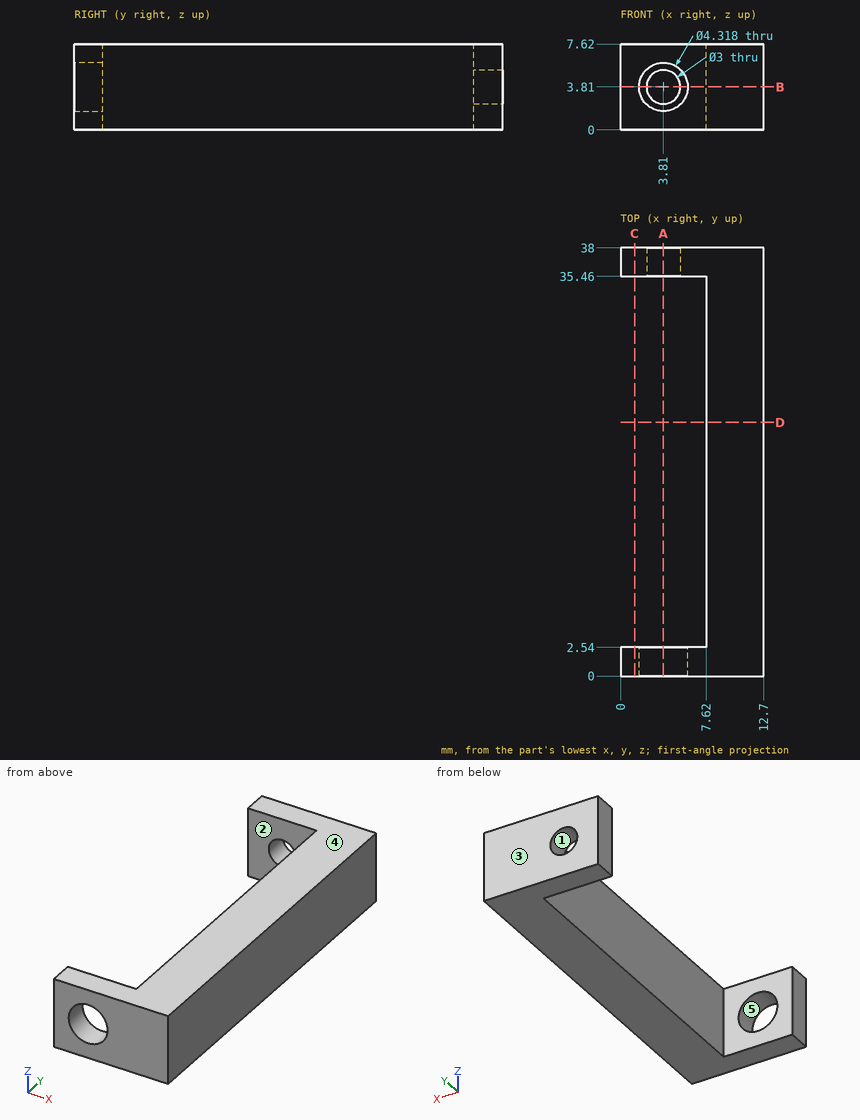
Input: dimensioned drawing with shaded views. Units: mm. Origin: part minimum x, y, z. A direction names the side the tool comes from. Coordinates: 2 decimals unless noted, no trailing zeros. Order: outer loops, then holes, each group sorted by start corner. A loop starts at its lowest first (then second) coordinate and runs counter-clockwise, first axis right, second up.
(1) Material intervals for probe 1 along Y at (x, z) = (0.5, 5.5); probe 2 along X at (y, z) = (1.4, 3.81); probe 3 along X at (y, z) = (31.5, 4), sorted ascending.
(2) Access query for the marked faces 1 and 2. Directions: +Z, -Z, +X, -X, +Y, -Y. A direction counts if a zero-diameter tool reaches every point of the face in a straight line with its end or side. Return the directions, or none.
(3) First-contact query: pin 1 (4 mm diameter, centred on y = 14.5, z = 3.5, fed in from -X); pin 2 (4 mm diameter, centred on x = 3.81, z = 3.81, fed in from -Y). Flat tips, straight axial feed; report the tip coordinate or a pass-through.
(4) Draft query along Z for the marked faces 3, 4 and 5. Return one class per face: pulls with the +Z half, pulls with the -Z half, needs draft (parallel to the pull), parting line crosses it, or undercut.
(5) Section query C-C (x = 1.25). Return the cut outline in (y, z), plus the area to 3 significant figures.
(6) Section query A-A (x = 3.81). Return the cut outline in (y, z).
(7) Section query D-D (y = 22.5). Return the cut outline in (x, z).
(8) Section query B-B (z = 3.81). Return the cut outline in (x, y), plus the area to 3 significant figures.
Solution:
1. probe 1: y = 0 to 2.54, 35.46 to 38
1. probe 2: x = 0 to 1.65, 5.97 to 12.7
1. probe 3: x = 7.62 to 12.7
2. face 1: +Y, -Y
2. face 2: +Z, -Z, -X
3. pin 1: stops at x = 7.62
3. pin 2: stops at y = 35.46
4. face 3: needs draft
4. face 4: pulls with the +Z half
4. face 5: undercut
5. outline: (0, 0) - (2.54, 0) - (2.54, 7.62) - (0, 7.62) - close; (35.46, 0) - (38, 0) - (38, 7.62) - (35.46, 7.62) - close
5. area: 38.7 mm2
6. outline: (0, 0) - (2.54, 0) - (2.54, 1.65) - (0, 1.65) - close; (0, 5.97) - (2.54, 5.97) - (2.54, 7.62) - (0, 7.62) - close; (35.46, 0) - (38, 0) - (38, 2.31) - (35.46, 2.31) - close; (35.46, 5.31) - (38, 5.31) - (38, 7.62) - (35.46, 7.62) - close
7. outline: (7.62, 0) - (12.7, 0) - (12.7, 7.62) - (7.62, 7.62) - close
8. outline: (0, 0) - (1.65, 0) - (1.65, 2.54) - (0, 2.54) - close; (0, 35.46) - (2.31, 35.46) - (2.31, 38) - (0, 38) - close; (5.31, 35.46) - (7.62, 35.46) - (7.62, 2.54) - (5.97, 2.54) - (5.97, 0) - (12.7, 0) - (12.7, 38) - (5.31, 38) - close
8. area: 213 mm2
